```python
from build123d import *

# Parameters (mm, degrees)
BOSS_EXTRUDE1_DEPTH       = 15
BOSS_EXTRUDE2_DEPTH       = 37.5
SKETCH8_R                 = 35
SKETCH8_R_2               = 18
BOSS_EXTRUDE13_DEPTH      = 100
CUT_EXTRUDE2_START        = -100
SKETCH13_R                = 18
CUT_EXTRUDE2_DEPTH        = 100
SKETCH14_R                = 18
SKETCH14_R_2              = 9
BOSS_EXTRUDE15_DEPTH      = 4
CUT_EXTRUDE3_START        = -50
SKETCH15_R                = 9
CUT_EXTRUDE3_DEPTH        = 50
BOSS_EXTRUDE16_REACH      = 249.48
BOSS_EXTRUDE16_END_RADIUS = 35
SKETCH18_R                = 24
SKETCH19_R                = 12.5
CUT_EXTRUDE4_DEPTH        = 50


with BuildPart() as part:
    # Sketch5 → Boss-Extrude1 (new body)
    with BuildSketch(Plane(origin=(0, 0, 0), x_dir=(1, 0, 0), z_dir=(0, 1, 0))):
        with BuildLine():
            Line((-37.5, -7.876252255), (-83.769584953, 64.123747745))
            ThreePointArc((-83.769584953, 64.123747745), (-84.643426785, 88.600912666), (-63.579244399, 101.098729377))
            Line((-63.579244399, 101.098729377), (-26.201026839, 101.098729377))
            ThreePointArc((-26.201026839, 101.098729377), (0, 112.630318244), (26.201026839, 101.098729377))
            Line((26.201026839, 101.098729377), (63.579244399, 101.098729377))
            ThreePointArc((63.579244399, 101.098729377), (84.643426785, 88.600912666), (83.769584953, 64.123747745))
            Line((83.769584953, 64.123747745), (37.5, -7.876252255))
            Line((37.5, -7.876252255), (-37.5, -7.876252255))
        make_face()
    extrude(amount=BOSS_EXTRUDE1_DEPTH)

    # Sketch7 → Boss-Extrude2 (add, symmetric)
    with BuildSketch(Plane(origin=(0, 0, 0), x_dir=(0, 0, -1), z_dir=(1, 0, 0))):
        with BuildLine():
            Line((-7.876252255, 0), (-63.876252255, 0))
            Line((-63.876252255, 0), (-63.876252255, 40.190310044))
            ThreePointArc((-63.876252255, 40.190310044), (-35.876252255, 68.190310044), (-7.876252255, 40.190310044))
            Line((-7.876252255, 40.190310044), (-7.876252255, 0))
        make_face()
    extrude(amount=BOSS_EXTRUDE2_DEPTH, both=True)

    # Sketch8 → Boss-Extrude13 (add)
    with BuildSketch(Plane(origin=(0, 15, 0), x_dir=(1, 0, 0), z_dir=(0, 1, 0))):
        with Locations(Location((0, 77.098729377, 0), (0, 0, 90))):
            Circle(SKETCH8_R)
        with Locations(Location((0, 77.098729377, 0), (0, 0, 90))):
            Circle(SKETCH8_R_2, mode=Mode.SUBTRACT)
    extrude(amount=BOSS_EXTRUDE13_DEPTH)

    # Sketch13 → Cut-Extrude2 (cut)
    with BuildSketch(Plane(origin=(0, 15, 0), x_dir=(1, 0, 0), z_dir=(0, 1, 0)).offset(CUT_EXTRUDE2_START)):
        with Locations(Location((0, 77.098729377, 0), (0, 0, 90))):
            Circle(SKETCH13_R)
    extrude(amount=CUT_EXTRUDE2_DEPTH, mode=Mode.SUBTRACT)

    # Sketch14 → Boss-Extrude15 (add)
    # profile 1 of 2: a face of its own
    with BuildSketch(Plane(origin=(0, 15, 0), x_dir=(1, 0, 0), z_dir=(0, 1, 0))):
        with Locations(Location((-63.579244399, 77.098729377, 0), (0, 0, 270))):
            Circle(SKETCH14_R)
        with Locations(Location((-63.579244399, 77.098729377, 0), (0, 0, 270))):
            Circle(SKETCH14_R_2, mode=Mode.SUBTRACT)
    # profile 2 of 2: a face of its own
    with BuildSketch(Plane(origin=(0, 15, 0), x_dir=(1, 0, 0), z_dir=(0, 1, 0))):
        with Locations(Location((63.579244399, 77.098729377, 0), (0, 0, 270))):
            Circle(SKETCH14_R)
        with Locations(Location((63.579244399, 77.098729377, 0), (0, 0, 270))):
            Circle(SKETCH14_R_2, mode=Mode.SUBTRACT)
    extrude(amount=BOSS_EXTRUDE15_DEPTH)

    # Sketch15 → Cut-Extrude3 (cut)
    with BuildSketch(Plane(origin=(0, 15, 0), x_dir=(1, 0, 0), z_dir=(0, 1, 0)).offset(CUT_EXTRUDE3_START)):
        with Locations(Location((-63.579244399, 77.098729377, 0), (0, 0, 270))):
            Circle(SKETCH15_R)
        with Locations(Location((63.579244399, 77.098729377, 0), (0, 0, 270))):
            Circle(SKETCH15_R)
    extrude(amount=CUT_EXTRUDE3_DEPTH, mode=Mode.SUBTRACT)

    # Boss-Extrude16: up to this cylinder (the profile starts outside it)
    boss_extrude16_end = Plane(origin=(0, 89, -77.098729377), z_dir=(0, -1, 0)) * Cylinder(BOSS_EXTRUDE16_END_RADIUS, 569.96, mode=Mode.PRIVATE)
    # Sketch18 → Boss-Extrude16 (add, up to the surface)
    with BuildSketch(Plane.XY.offset(-137), mode=Mode.PRIVATE) as boss_extrude16_sk1:
        with Locations(Location((0, 89, 0), (0, 0, 90))):
            Circle(SKETCH18_R)
    boss_extrude16_tool1 = extrude(boss_extrude16_sk1.sketch, amount=BOSS_EXTRUDE16_REACH, mode=Mode.PRIVATE) - boss_extrude16_end
    add(boss_extrude16_tool1.solids().sort_by_distance((0, 89, -137))[0])

    # Sketch19 → Cut-Extrude4 (cut)
    with BuildSketch(Plane(origin=(0, 0, -137), x_dir=(-1, 0, 0), z_dir=(0, 0, -1))):
        with Locations((0, 89)):
            Circle(SKETCH19_R)
    extrude(amount=-CUT_EXTRUDE4_DEPTH, mode=Mode.SUBTRACT)


solid = part.part
```
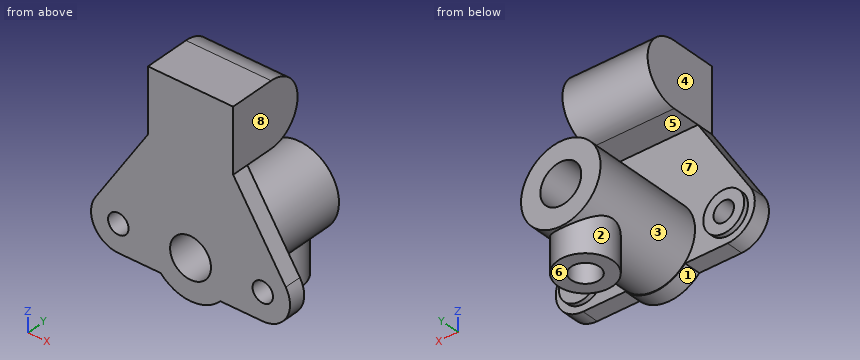
Here's how the part is built. I have some questions about the finished solid (model axes, mm). Face numbers are marked on the shaded views. A direction names the side the tool comes from. Give positions to 0.01 mm unless a question says otherwise; leave off trailing zeros. Write each loop counter-clockwise with the first axis right and the second up, starting at its lowest first coordinate (ties: lowest second). Pieces come first, ordered by that corner, then holes.
(1) Imagine slicing it at C-C, the plane y = 89. Write out the boundary of the cut face in (x, z).
Output values:
outline: (-24, -137) - (-12.5, -137) - (-12.5, -90.05) arc R18 cw (long way) to (12.5, -90.05) - (12.5, -137) - (24, -137) - (24, -102.57) arc R35 ccw (long way) to (-24, -102.57) - close
(2) Imagine slicing it at D-D, the plane z = -124. Write out the boundary of the cut face in (x, y), and give its area (3 significant figures).
Output values:
outline: circle Ø48 at (0, 89); hole circle Ø25 at (0, 89)
area: 1,320 mm2
(3) Imagine slicing it at A-A, the plane x = 0. Write out the boundary of the cut face in (y, z).
Output values:
outline: (0, -112.63) - (15, -112.63) - (15, -112.1) - (65, -112.1) - (65, -137) - (76.5, -137) - (76.5, -95.1) - (0, -95.1) - close; (0, -59.1) - (115, -59.1) - (115, -42.1) - (15, -42.1) - (15, 7.88) - (40.19, 7.88) arc R28 ccw to (40.19, 63.88) - (0, 63.88) - close; (101.5, -137) - (113, -137) - (113, -112.1) - (115, -112.1) - (115, -95.1) - (101.5, -95.1) - close
(4) Imagine slicing it at B-B, the plane y = 36. Write out the boundary of the cut face in (x, z).
Output values:
outline: (-37.5, 7.88) - (37.5, 7.88) - (37.5, 63.88) - (-37.5, 63.88) - close; circle Ø70 at (0, -77.1); hole circle Ø36 at (0, -77.1)
(5) On a 3-axis mill with a long thin cutter (end or side, diameter ignored), from which of +Z, -Z, +X, -X, +Y, -Y can I reach the whole of each face in a straight line? I mean the marked faces 1, 2, 3 and 4. Say none if no direction works.
Output values:
face 1: -Z, -Y
face 2: -Z
face 3: none
face 4: +Z, -X, +Y, -Y
(6) Thinking about a two-plate mould opening in Z: for the marked faces 5, 6, 7 and 8, which applies, pulls with the +Z half, pulls with the -Z half, needs draft (parallel to the pull), parting line crosses it, or undercut?
Output values:
face 5: undercut
face 6: pulls with the -Z half
face 7: undercut
face 8: needs draft
(7) Will these pins go through, and if not, where does the flat tip stop? pin 1 (5 mm diameter, centred on y = 46, z = -58.5, fed in from -X); pin 2 (16.5 mm diameter, centred on x = 53, y = 9.5, fed in from -Z); pin 3 (20 mm diameter, centred on x = 18, y = 31, fed in from -Z).
Output values:
pin 1: stops at x = -31.08
pin 2: stops at z = -101.1
pin 3: stops at z = -111.17
(8) If I drill on L1, parallel to Z at x = -9, y = 61.5; L2, parallel to Z at x = 58, y = 16.5; L3, parallel to Y at x = 1, z = -110, over which ranges is the centre line in solid material (lowest first)?
Output values:
L1: z = -110.92 to -92.69, -61.51 to -43.28, 17.71 to 54.04
L2: z = -94.21 to -84.16, -70.04 to -59.99
L3: y = 0 to 76.54, 101.46 to 115
